For this review, take the finished solid that the model builds, in its own axes (mm). Face numbers are marked on the shaded views. Coordinates: 2 decimals unless noted, no trailing zeros. Loops run counter-clockwise (first coordinate to the right, second up) from the corner with the lowest first, then second, coordinate; pieces in that order, holes last. Notation, with made-up numbers: M 88.25,62 L 102.25,62 A20 cw 102.25,73 Z; hole C 41.25,9 d6. An arc over 180 degrees is marked long. Answer as a JSON object with one key per item and string values. Group by question number.
Item 1: Add section C-C (z = 4). State the section outline as (x, y) points, then the cut area to 3 significant figures.
Item 2: Insertion check: pin 1 (5 mm diameter, centred on x = -0.5, y = 4.5, fed in from -Z); pin 2 (6 mm diameter, centred on y = 4, z = 0.5, fed in from -X) (3 decimals); pin 3 (6 mm diameter, centred on y = 4.5, z = 3.5, fed in from +X); pin 4 (1.5 mm diameter, centred on y = 1, z = 4, fed in from +X). Each pin has a flat end and moves straight along its axis. Give the tip position at first contact, or say it passes through.
Item 3: Wall thickness on L1, parallel to Y at x = 0, z = -3.5; L2, parallel to Z at x = 1, y = 7.75; L3, parallel to X at y = 3.5, z = 6.5: over which ranges is each line inside the solid? List them lowest first. Write a range as from..to.
Item 4: Mouldability with a two-part tool opening along Y and no side actions: class the marked faces 1 and 2 as +Y half, -Y half, draft (parallel to the pull), parting line (faces both ways), or undercut.
Item 5: Add section D-D (z = -5.5). State the section outline as (x, y) points.
Item 6: Add section A-A (y = 0). State the section outline as (x, z) points, then the cut area to 3 significant figures.
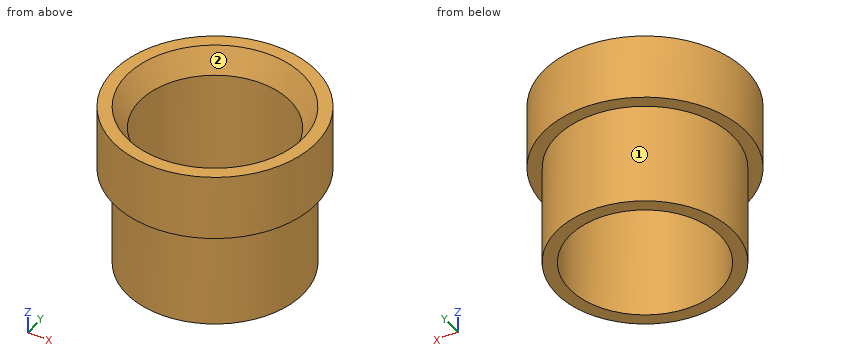
from build123d import *


with BuildPart() as part:
    # Sketch1 → Revolve1 (revolve)
    with BuildSketch(Plane(origin=(0, 0, 0), x_dir=(0, 0, -1), z_dir=(1, 0, 0)), mode=Mode.PRIVATE) as revolve1_sk:
        Polygon((-7.112, 7.52475), (-5.18725854, 6.4135), (7.112, 6.4135), (7.112, 7.52475), (-1.524, 7.52475), (-1.524, 8.636), (-7.112, 8.636), align=None)
    revolve(revolve1_sk.sketch.rotate(Axis((0, 0, -7.112), (0, 0, 1)), 90), axis=Axis((0, 0, -7.112), (0, 0, 1)))


solid = part.part
From the geometry:
{
 "1": {"outline": "C 0,0 d17.27; hole C 0,0 d12.83", "area": "105 mm²"},
 "2": {"pin 1": "stops at z = -7.11", "pin 2": "stops at x = -8.555", "pin 3": "stops at x = 8.5", "pin 4": "stops at x = 8.63"},
 "3": {"L1": "y = -7.52..-6.41, 6.41..7.52", "L2": "z = 1.52..7.11", "L3": "x = -7.89..-6.26, 6.26..7.89"},
 "4": {"face 1": "parting line", "face 2": "undercut"},
 "5": {"outline": "C 0,0 d15.05; hole C 0,0 d12.83"},
 "6": {"outline": "M -8.64,1.52 L -7.52,1.52 L -7.52,-7.11 L -6.41,-7.11 L -6.41,5.19 L -7.52,7.11 L -8.64,7.11 Z; M 6.41,-7.11 L 7.52,-7.11 L 7.52,1.52 L 8.64,1.52 L 8.64,7.11 L 7.52,7.11 L 6.41,5.19 Z", "area": "41.9 mm²"}
}
